```python
from build123d import *

# Parameters (mm, degrees)
EXTRUDE_1_DEPTH     = 4
SKETCH_2_R          = 1.5
SKETCH_2_R_2        = 2
SKETCH_2_W          = 4.4
SKETCH_2_H          = 8.4
CUT_EXTRUDE_1_DEPTH = 4
SKETCH_3_W          = 87
SKETCH_3_H          = 3.5
EXTRUDE_2_DEPTH     = 4


with BuildPart() as part:
    # 草图1 → 凸台-拉伸1 (new body)
    with BuildSketch(Plane.XY):
        Polygon((37.5, 50), (-37.5, 50), (-43.5, 50), (-43.5, -57), (-43.5, -164), (-37.5, -164), (37.5, -164), (43.5, -164), (43.5, -57), (43.5, 50), align=None)
        Polygon((-29.5, -156), (-29.5, -94.879730583), (20.598581489, -156), align=None, mode=Mode.SUBTRACT)
        Polygon((-20.598581489, -80.5), (29.5, -80.5), (29.5, -141.620269417), align=None, mode=Mode.SUBTRACT)
        with BuildLine():
            ThreePointArc((-19.08974359, -49.021094412), (0, -33.5), (19.08974359, -49.021094412))
            ThreePointArc((19.08974359, -49.021094412), (23.5, -53), (19.08974359, -56.978905588))
            ThreePointArc((19.08974359, -56.978905588), (0, -72.5), (-19.08974359, -56.978905588))
            ThreePointArc((-19.08974359, -56.978905588), (-23.5, -53), (-19.08974359, -49.021094412))
        make_face(mode=Mode.SUBTRACT)
        Polygon((-29.5, 42), (19.561080579, 42), (-29.5, -12.621336377), align=None, mode=Mode.SUBTRACT)
        Polygon((-19.561080579, -25.5), (29.5, 29.121336377), (29.5, -25.5), align=None, mode=Mode.SUBTRACT)
    extrude(amount=EXTRUDE_1_DEPTH)

    # 草图2 → 切除-拉伸1 (cut)
    with BuildSketch(Plane.XY.offset(4)):
        with Locations((37.5, -158)):
            Circle(SKETCH_2_R)
        with Locations((37.5, -78)):
            Circle(SKETCH_2_R)
        with Locations((37.5, -118)):
            Circle(SKETCH_2_R)
        with Locations((37.5, 44)):
            Circle(SKETCH_2_R_2)
        with Locations((-37.5, 44)):
            Circle(SKETCH_2_R_2)
        with Locations((-37.5, -41)):
            Circle(SKETCH_2_R_2)
        with Locations((-37.5, -126)):
            Circle(SKETCH_2_R_2)
        with Locations((37.5, -138)):
            Rectangle(SKETCH_2_W, SKETCH_2_H)
        with Locations((37.5, -98)):
            Rectangle(SKETCH_2_W, SKETCH_2_H)
        with Locations((37.5, -58)):
            Rectangle(SKETCH_2_W, SKETCH_2_H)
    extrude(amount=-CUT_EXTRUDE_1_DEPTH, mode=Mode.SUBTRACT)

    # 草图3 → 凸台-拉伸2 (add)
    with BuildSketch(Plane.XY.offset(4)):
        with Locations((0, -165.75)):
            Rectangle(SKETCH_3_W, SKETCH_3_H)
    extrude(amount=-EXTRUDE_2_DEPTH)


solid = part.part
```
Here's how the part is built. I have some questions about the finished solid (model axes, mm). A direction names the side the tool comes from. Coordinates: 2 decimals unless noted, no trailing zeros. Order: outer loops, then holes, each group sorted by start corner. A loop starts at its lowest first (then second) coordinate and runs counter-clockwise, first axis right, second up.
1) Imagine slicing it at C-C on y = -126. List the corners of the cut face in (x, z) for me, and give its area (3 significant figures).
2) Imagine slicing it at B-B on y = -68. List the corners of the cut face in (x, z) for me.
3) Imagine slicing it at D-D on x = 7. List the corners of the cut face in (y, z) for me, and give its area (3 significant figures).
4) Imagine slicing it at A-A on x = -37.5. List the corners of the cut face in (y, z) for me, and give its area (3 significant figures).
5) Which directions (+Z, -Z, +X, -X, +Y, -Y) give clear straight access to the entire face, cutting with the end or side of a thin tool? Please do faces 1 (the face through (-19.9, -57.2, 4)), 2 (the face through (37, -102.2, 2)).
6) We'd pull the mould along Y, two halves only. Please class faces 3 (the face through (-43.5, -60, 2)), 4 (the face through (-0.373, -33.504, 1.972)), 5 (the face through (1, 50, 2)): +Y half, -Y half, draft (parallel to the pull), parting line (faces both ways), or undercut.
7) I need wall thicknesses on line 1 (X direction, y = -53, z = 2.6); line 2 (Y direction, x = -27.5, z = 2.35); line 3 (Y direction, x = 16, z = 1.9). Which ranges of each line are inside material? Lowest first, please.
Response values:
1. outline: (-43.5, 0) - (-39.5, 0) - (-39.5, 4) - (-43.5, 4) - close; (-35.5, 0) - (-29.5, 0) - (-29.5, 4) - (-35.5, 4) - close; (-3.99, 0) - (16.7, 0) - (16.7, 4) - (-3.99, 4) - close; (29.5, 0) - (43.5, 0) - (43.5, 4) - (29.5, 4) - close
1. area: 179 mm2
2. outline: (-43.5, 0) - (-12.46, 0) - (-12.46, 4) - (-43.5, 4) - close; (12.46, 0) - (43.5, 0) - (43.5, 4) - (12.46, 4) - close
3. outline: (-167.5, 0) - (-156, 0) - (-156, 4) - (-167.5, 4) - close; (-139.41, 0) - (-114.17, 0) - (-114.17, 4) - (-139.41, 4) - close; (-80.5, 0) - (-71.2, 0) - (-71.2, 4) - (-80.5, 4) - close; (-34.8, 0) - (-25.5, 0) - (-25.5, 4) - (-34.8, 4) - close; (4.07, 0) - (28.02, 0) - (28.02, 4) - (4.07, 4) - close; (42, 0) - (50, 0) - (50, 4) - (42, 4) - close
3. area: 349 mm2
4. outline: (-167.5, 0) - (-128, 0) - (-128, 4) - (-167.5, 4) - close; (-124, 0) - (-43, 0) - (-43, 4) - (-124, 4) - close; (-39, 0) - (42, 0) - (42, 4) - (-39, 4) - close; (46, 0) - (50, 0) - (50, 4) - (46, 4) - close
4. area: 822 mm2
5. face 1: +Z, +X, -X, +Y, -Y
5. face 2: +Z, -Z
6. face 3: draft
6. face 4: undercut
6. face 5: +Y half
7. line 1: x = -43.5 to -23.5, 23.5 to 43.5
7. line 2: y = -167.5 to -156, -97.32 to -10.39, 42 to 50
7. line 3: y = -167.5 to -156, -150.39 to -125.15, -80.5 to -64.15, -41.85 to -25.5, 14.09 to 38.04, 42 to 50
